Autodesk Inventor part; units mm, degrees
ref_plane "YZ Plane" through (0, 0, 0) normal (1, 0, 0) x (0, 1, 0)
ref_plane "XZ Plane" through (0, 0, 0) normal (0, 1, 0) x (-1, 0, 0)
ref_plane "XY Plane" through (0, 0, 0) normal (0, 0, 1) x (1, 0, 0)
sketch "Sketch1" plane through (0, 0, 0) normal (0, 0, 1) x (1, 0, 0)
  line L0 (2.0907, -12.7904) -> (2.0907, 12.2096)
  line L1 (2.0907, 12.2096) -> (-15.9093, 12.2096)
  line L2 (-15.9093, 12.2096) -> (-15.9093, -12.7904)
  line L3 (-15.9093, -12.7904) -> (2.0907, -12.7904)
  line L4 (-15.9093, 17.2096) -> (-15.9093, -14.7904) construction
  line L5 (2.0907, -14.7904) -> (2.0907, 17.2096) construction
  dimension "d27" = 25
extrude "Extrusion1" add sketch "Sketch1" along normal blind 2
sketch "Sketch2" plane through (-15.9093, -7.7904, 0) normal (-1, 0, 0) x (0, 0, 1)
  circle A0 centre (5.7, -0.7) radius 1.25 construction
  line L0 (2, -5) -> (6.216, -4.4143)
  arc A1 (6.216, -4.4143) -> (6.216, 3.0143) centre (5.7, -0.7) ccw
  line L1 (5.7, -0.7) -> (2, -0.7) construction
  line L2 (2, 3.6) -> (6.216, 3.0143)
  line L3 (2, 3.6) -> (2, -5)
  line L4 (0, -5) -> (2, -5) construction
  arc A2 (4.4, -0.7) -> (7, -0.7) centre (5.7, -0.7) ccw construction
  dimension "d2" = 2.5
  dimension "d3" = 3.75
extrude "Extrusion2" add sketch "Sketch2" against normal blind 3
ref_plane "Work Plane1" through (-6.9093, -12.7904, 0) normal (-1, 0, 0) x (0, 0, 1)
mirror "Mirror1" about plane through (-6.9093, -12.7904, 0) normal (-1, 0, 0) of "Extrusion2"
hole "Hole1" at (-15.9093, -8.4904, 5.7) direction (1, 0, 0) diameter 2.6 end through all
sketch "Sketch3" plane through (-0.9093, -8.4904, 5.7) normal (-1, 0, 0) x (0, 0, 1)
  circle A0 centre (0, 0) radius 1.3
  line L0 (-1.4722, -2.55) -> (-2.9445, 0)
  line L1 (-2.9445, 0) -> (-1.4722, 2.55)
  line L2 (-1.4722, 2.55) -> (1.4722, 2.55)
  line L3 (1.4722, 2.55) -> (2.9445, 0)
  line L4 (2.9445, 0) -> (1.4722, -2.55)
  line L5 (1.4722, -2.55) -> (-1.4722, -2.55)
  point P0 (-5.7, 8.4904)
  point P1 (0, 0)
  dimension "d18" = 5.1
extrude "Extrusion3" cut sketch "Sketch3" against normal blind 2.1
sketch "Sketch4" plane through (-15.9093, -12.7904, 0) normal (-1, 0, 0) x (0, 0, 1)
  arc A0 (5.3473, 20.4706) -> (5.3473, 24.4098) centre (5, 22.4402) ccw
  line L0 (5, 22.4402) -> (2, 22.4402) construction
  line L1 (2, 25) -> (2, 8.6) construction
  line L2 (5.3473, 24.4098) -> (2, 25)
  line L3 (5.3473, 20.4706) -> (2, 19.8803)
  line L4 (2, 25) -> (2, 19.8803)
  point P0 (0, 12.7904)
  dimension "d21" = 2
  dimension "d22" = 3
  dimension "d24" = 80
extrude "Extrusion4" add sketch "Sketch4" against normal up to surface (18 mm away)
thicken "Thicken1" operation add thickness 0.1 both sides no extend neighbours yes toward (-1, 0, 0) faces at (2.0907, -1.5904, 0.6667)
thicken "Thicken2" operation add thickness 0.1 both sides no extend neighbours yes toward (0, 0, 1) faces at (-3.976, -4.4571, 0)
properties part number "Encoder_Mount1_Slider"
Geometry check sheet. Reference: the model listing, model coordinates, mm. A direction names the side the tool comes from. Give positions to 0.01 mm unless a question says otherwise; leave off trailing zeros. Order: outer loops, then holes, each group sorted by start corner. A loop starts at its lowest first (then second) coordinate and runs counter-clockwise, first axis right, second up. Notation, with made-up numbers: (56.5, -17.5) - (79.5, -17.5) arc R31 cw to (79.5, 13.5) - close; hole circle Ø1 at (74.25, -18). An arc over 180 degrees is marked (long way). Answer in a Markdown table with one row per item. Add a question column.
Q1. Gauge pin test, flat ends, axial feed: pin 1 (1.5 mm diameter, centred on x = -2, z = 5.5, fed in from -Y); pin 2 (2.5 mm diameter, centred on y = -9.5, z = 5.5, fed in from -X); pin 3 (0.6 mm diameter, centred on x = 0, z = 6, fed in from +Y); pin 4 (1 mm diameter, centred on x = -7, z = 6.5, fed in from -Y). Record the tip position at first contact, or that the pin passes through.
Q2. Tool access check on faces 1 (the flat face through (-7.08, 7.39, 3.7)), 2 (the flat face through (-0.909, -7, 3)), 3 (the flat face through (0, -11.04, 6)). Record the directions out of +Z, -Z, +X, -X, +Y, -Y that give a thin tool (end or side, any length) a straight path to the whole face; none if there is none.
Q3. Mould release check, pull along Y, two halves, no side actions. Record for faces 4 (the flat face through (-7, -12.79, 1)), 5 (the flat face through (-7, -3, 2)), 6 (the flat face through (-7, 12.21, 1)), 7 (the flat face through (-14.43, -4.48, 4.08)): pulls with the +Y half, pulls with the -Y half, needs draft (parallel to the pull), parting line crosses it, or undercut.
Q4. Cross-section at C-C, the plane z = 3.5. Enter the section's corners in (x, y), then the cut area to 3 significant figures.
Q5. Cross-section at D-D, the plane y = 0. Enter the section's corners in (x, z), then the cut area to 3 significant figures.
Q6. Material ranges on probe 1 along X at (y, z) = (-7.75, 7); probe 2 along Y at (x, z) = (1.8, 5.7); probe 3 along Z at (x, y) = (-11.25, -7.75), recorded low to high. Write a range as from..to.
Q7. Cross-section at A-A, the plane z = 5.7. Enter the section's corners in (x, y).
Q8. Cross-section at B-B, the plane x = -12.5. Enter the section's corners in (y, z), then the cut area to 3 significant figures.
Check values:
| question | item | result |
|---|---|---|
| 1 | pin 1 | stops at y = 7.57 |
| 1 | pin 2 | stops at x = -15.91 |
| 1 | pin 3 | stops at y = 11.52 |
| 1 | pin 4 | stops at y = 7.92 |
| 2 | face 1 | +Z, +X, -X |
| 2 | face 2 | +Z, -Y |
| 2 | face 3 | none |
| 3 | face 4 | pulls with the -Y half |
| 3 | face 5 | undercut |
| 3 | face 6 | pulls with the +Y half |
| 3 | face 7 | undercut |
| 4 | outline | (-15.91, -12.58) - (-12.91, -12.58) - (-12.91, -4.4) - (-15.91, -4.4) - close; (-15.91, 7.35) - (1.99, 7.35) - (1.99, 11.95) - (-15.91, 11.95) - close; (-0.91, -12.58) - (1.99, -12.58) - (1.99, -4.4) - (-0.91, -4.4) - (-0.91, -7.2) - (1.19, -7.2) - (1.19, -9.78) - (-0.91, -9.78) - close |
| 4 | area | 125 mm^2 |
| 5 | outline | (-15.91, 0.1) - (1.99, 0.1) - (1.99, 2) - (-15.91, 2) - close |
| 5 | area | 34.0 mm^2 |
| 6 | probe 1 | x = -15.91..-12.91, 1.19..1.99 |
| 6 | probe 2 | y = -12.28..-9.79, -7.19..-4.7, 7.78..11.52 |
| 6 | probe 3 | z = 0.1..2 |
| 7 | outline | (-15.91, -12.28) - (-12.91, -12.28) - (-12.91, -9.79) - (-15.91, -9.79) - close; (-15.91, -7.19) - (-12.91, -7.19) - (-12.91, -4.7) - (-15.91, -4.7) - close; (-15.91, 7.78) - (1.99, 7.78) - (1.99, 11.52) - (-15.91, 11.52) - close; (-0.91, -12.28) - (1.99, -12.28) - (1.99, -9.79) - (1.19, -9.79) - (1.19, -11.04) - (-0.91, -11.04) - close; (-0.91, -5.94) - (1.19, -5.94) - (1.19, -7.19) - (1.99, -7.19) - (1.99, -4.7) - (-0.91, -4.7) - close |
| 8 | outline | (-12.79, 0.1) - (12.21, 0.1) - (12.21, 2) - (11.62, 5.35) arc R2 ccw to (7.68, 5.35) - (7.09, 2) - (-12.79, 2) - close |
| 8 | area | 67.6 mm^2 |
